Geometry: final body of the model. Coordinates: model frame, mm. A direction names the side the tool comes from. Give positions to 0.01 mm unless a question says otherwise; leave off trailing zeros. Loops run counter-clockwise (first coordinate to the right, second up) from the corner with the lowest first, then second, coordinate; pieces in that order, holes last. Notation, with made-up numbers: (-21, 38.5) -> (25, 38.5) arc R27 cw to (25, 77.5) -> close; hole circle Ø8 at (3.5, 55.5). An arc over 180 degrees is marked (long way). Answer in a Markdown table with one row per item. Add a question column.
from build123d import *

# Parameters (mm, degrees)
F0_W     = 20.32
F0_H     = 20.32
F0_W_2   = 15.24
F0_H_2   = 15.24
F1_DEPTH = 3.81
F2_DEPTH = 17.78
F3_R     = 4.064
F4_DEPTH = 25.4
F5_R     = 1.27
F6_R     = 0.508


with BuildPart() as f1:
    # F0 (on Top) → F1 (new body)
    with BuildSketch(Plane.XY):
        Rectangle(F0_W, F0_H)
        Rectangle(F0_W_2, F0_H_2, mode=Mode.SUBTRACT)
        Rectangle(F0_W_2, F0_H_2)
    extrude(amount=F1_DEPTH)

    # F0 (on Top) → F2 (join)
    with BuildSketch(Plane.XY):
        Rectangle(F0_W, F0_H)
        Rectangle(F0_W_2, F0_H_2, mode=Mode.SUBTRACT)
    extrude(amount=-F2_DEPTH)

    # F3 (on Top) → F4 (cut)
    with BuildSketch(Plane.XY):
        Circle(F3_R)
    extrude(amount=F4_DEPTH, mode=Mode.SUBTRACT)

    # F5
    f5_edges = [f1.edges().sort_by_distance(p)[0] for p in [
        (-10.16, 0, 3.81),
        (0, 10.16, 3.81),
        (10.16, 0, 3.81),
        (0, -10.16, 3.81),
        (-10.16, 10.16, -6.985),
        (-10.16, -10.16, -6.985),
        (-10.16, 0, -17.78),
        (10.16, 10.16, -6.985),
        (10.16, 0, -17.78),
        (10.16, -10.16, -6.985),
        (0, -10.16, -17.78),
        (0, 10.16, -17.78),
    ]]
    fillet(f5_edges, radius=F5_R)

    # F6
    f6_edges = [f1.edges().sort_by_distance(p)[0] for p in [
        (-7.62, -7.62, -8.89),
        (7.62, -7.62, -8.89),
        (7.62, 7.62, -8.89),
        (-7.62, 7.62, -8.89),
    ]]
    fillet(f6_edges, radius=F6_R)


solid = f1.part
(1) Reachability of faces 5 (the flat face through (0, -7.62, -9)), 6 (the cylindrical face through (0.124, -9.798, 3.428)) from +Z, -Z, +X, -X, +Y, -Y: full face, straight path, thin tool, end or side. Return the list, or none.
(2) Cut plane A-A on y = 0. Return the cut outline in (x, z), then the cut area to 3 significant figures.
(3) Material intervals for line 1 along X through (y, z) = (0, 0.9); line 2 along Y through (x, z) = (7, -8.5), sorted ascending. Write a range as from..to.
(4) Cut plane D-D on x = 6.25. Return the cut outline in (y, z), then the cut area to 3 significant figures.
(5) Cut plane B-B on z = -10.25. Return the cut outline in (x, y).
(6) Pin query (flat end, axial travel): pin 1 Ø4.5 at (x, y) = (1.5, 3.5) entering from -Z. Return the tip coordinate at first contact, or that it passes through.
(7) Draft query along X for faces 1 (the flat face through (10.16, 0, -7)), 2 (the cylindrical face through (0.124, -9.798, -17.398)), 3 (the cylindrical face through (-9.798, 0.124, -17.398)), 4 (the flat face through (0, 7.62, -9)). Return one class per face: +X half, -X half, draft (parallel to the pull), parting line (faces both ways), or undercut.
Answer list:
| question | item | result |
|---|---|---|
| 1 | face 5 | -Z |
| 1 | face 6 | +Z, +X, -X, -Y |
| 2 | outline | (-10.16, -16.51) arc R1.27 ccw to (-8.89, -17.78) -> (-7.62, -17.78) -> (-7.62, 0) -> (-4.06, 0) -> (-4.06, 3.81) -> (-8.89, 3.81) arc R1.27 ccw to (-10.16, 2.54) -> close; (4.06, 0) -> (7.62, 0) -> (7.62, -17.78) -> (8.89, -17.78) arc R1.27 ccw to (10.16, -16.51) -> (10.16, 2.54) arc R1.27 ccw to (8.89, 3.81) -> (4.06, 3.81) -> close |
| 2 | area | 135 mm² |
| 3 | line 1 | x = -10.16..-4.06, 4.06..10.16 |
| 3 | line 2 | y = -10.16..-7.62, 7.62..10.16 |
| 4 | outline | (-10.16, -16.51) arc R1.27 ccw to (-8.89, -17.78) -> (-7.62, -17.78) -> (-7.62, 0) -> (7.62, 0) -> (7.62, -17.78) -> (8.89, -17.78) arc R1.27 ccw to (10.16, -16.51) -> (10.16, 2.54) arc R1.27 ccw to (8.89, 3.81) -> (-8.89, 3.81) arc R1.27 ccw to (-10.16, 2.54) -> close |
| 4 | area | 166 mm² |
| 5 | outline | (-10.16, -8.89) arc R1.27 ccw to (-8.89, -10.16) -> (8.89, -10.16) arc R1.27 ccw to (10.16, -8.89) -> (10.16, 8.89) arc R1.27 ccw to (8.89, 10.16) -> (-8.89, 10.16) arc R1.27 ccw to (-10.16, 8.89) -> close; hole (-7.62, -7.11) arc R0.51 ccw to (-7.11, -7.62) -> (7.11, -7.62) arc R0.51 ccw to (7.62, -7.11) -> (7.62, 7.11) arc R0.51 ccw to (7.11, 7.62) -> (-7.11, 7.62) arc R0.51 ccw to (-7.62, 7.11) -> close |
| 6 | pin 1 | stops at z = 0 |
| 7 | face 1 | +X half |
| 7 | face 2 | draft |
| 7 | face 3 | -X half |
| 7 | face 4 | undercut |
